from build123d import *

# Parameters (mm, degrees)
F0_W         = 70
F0_H         = 45
F0_W_2       = 20.7
F0_H_2       = 27.2
F0_W_3       = 25.5
F0_H_3       = 32.8
F1_DEPTH     = 2
F2_W         = 70
F2_H         = 45
F2_W_2       = 65
F2_H_2       = 40
F3_DEPTH     = 55
F4_W         = 70
F4_H         = 45
F4_W_2       = 13.2
F4_H_2       = 19.6
F5_DEPTH     = 2.5
F6_W         = 5
F6_H         = 2.5
F7_DEPTH     = 59.501
F8_T1_DEPTH  = 64
F8_T3_DEPTH  = 49.5
F8_T5_DEPTH  = 53.5
F8_S9_W      = 3
F8_S9_H      = 3
F8_T10_DEPTH = 3
F8_S15_W     = 3
F8_S15_H     = 3
F8_T16_DEPTH = 3
F8_S21_W     = 3
F8_S21_H     = 3
F8_T22_DEPTH = 3
F8_S27_W     = 3
F8_S27_H     = 3
F8_T28_DEPTH = 3


# Not quite as in the source:
# - a fillet or chamfer that OpenCascade refuses, or shapes differently, is made with other operations: its cross-section is extruded or revolved along the edge and cut away or added


with BuildPart() as f1:
    # F0 (on Front) → F1 (new body)
    with BuildSketch(Plane.XZ):
        Rectangle(F0_W, F0_H)
        with Locations((17.65, -1.9)):
            Rectangle(F0_W_2, F0_H_2, mode=Mode.SUBTRACT)
        with Locations((-15.25, 0.9)):
            Rectangle(F0_W_3, F0_H_3, mode=Mode.SUBTRACT)
    extrude(amount=F1_DEPTH)

    # F2 (on face) → F3 (join)
    with BuildSketch(Plane.XZ.offset(2)):
        Rectangle(F2_W, F2_H)
        Rectangle(F2_W_2, F2_H_2, mode=Mode.SUBTRACT)
    extrude(amount=F3_DEPTH)

    # F4 (on face) → F5 (join)
    with BuildSketch(Plane.XZ.offset(57)):
        Rectangle(F4_W, F4_H)
        Rectangle(F4_W_2, F4_H_2, mode=Mode.SUBTRACT)
    extrude(amount=F5_DEPTH)

    # F6 (on face) → F7 (cut, through all)
    with BuildSketch(Plane(origin=(0, 0, 0), x_dir=(-1, 0, 0), z_dir=(0, 1, 0))):
        with Locations((-30, -18.75)):
            Rectangle(F6_W, F6_H)
        with Locations((30, -18.75)):
            Rectangle(F6_W, F6_H)
    extrude(amount=-F7_DEPTH, mode=Mode.SUBTRACT)

    # F8: fillet of radius 3 on 8 edges, made by hand

    # F8_s2 → F8_t1 (cut)
    with BuildSketch(Plane.YZ.offset(-32)):
        with BuildLine():
            ThreePointArc((-56.5, 22.5), (-58.6213203436, 21.6213203436), (-59.5, 19.5))
            Line((-59.5, 19.5), (-59.5, 22.5))
            Line((-59.5, 22.5), (-56.5, 22.5))
        make_face()
        with BuildLine():
            ThreePointArc((-3, 22.5), (-0.8786796564, 21.6213203436), (0, 19.5))
            Line((0, 19.5), (0, 22.5))
            Line((0, 22.5), (-3, 22.5))
        make_face()
    extrude(amount=F8_T1_DEPTH, mode=Mode.SUBTRACT)

    # F8_s4 → F8_t3 (cut)
    with BuildSketch(Plane.XY.offset(-30)):
        with BuildLine():
            ThreePointArc((32, -59.5), (34.1213203436, -58.6213203436), (35, -56.5))
            Line((35, -56.5), (35, -59.5))
            Line((35, -59.5), (32, -59.5))
        make_face()
        with BuildLine():
            ThreePointArc((-35, -56.5), (-34.1213203436, -58.6213203436), (-32, -59.5))
            Line((-32, -59.5), (-35, -59.5))
            Line((-35, -59.5), (-35, -56.5))
        make_face()
        with BuildLine():
            ThreePointArc((32, 0), (34.1213203436, -0.8786796564), (35, -3))
            Line((35, -3), (35, 0))
            Line((35, 0), (32, 0))
        make_face()
        with BuildLine():
            ThreePointArc((-32, 0), (-34.1213203436, -0.8786796564), (-35, -3))
            Line((-35, -3), (-35, 0))
            Line((-35, 0), (-32, 0))
        make_face()
    extrude(amount=F8_T3_DEPTH, mode=Mode.SUBTRACT)

    # F8_s6 → F8_t5 (cut)
    with BuildSketch(Plane.XZ.offset(3)):
        with BuildLine():
            ThreePointArc((32, 22.5), (34.1213203436, 21.6213203436), (35, 19.5))
            Line((35, 19.5), (35, 22.5))
            Line((35, 22.5), (32, 22.5))
        make_face()
        with BuildLine():
            ThreePointArc((-32, 22.5), (-34.1213203436, 21.6213203436), (-35, 19.5))
            Line((-35, 19.5), (-35, 22.5))
            Line((-35, 22.5), (-32, 22.5))
        make_face()
    extrude(amount=F8_T5_DEPTH, mode=Mode.SUBTRACT)


with BuildPart() as f8_tool8:
    # F8_s9 → F8_t10 (new body)
    with BuildSketch(Plane.XY.offset(19.5)):
        with Locations((33.5, -58)):
            Rectangle(F8_S9_W, F8_S9_H)
    extrude(amount=F8_T10_DEPTH)

    # F8_s11 → F8_t12 (revolve, cut)
    with BuildSketch(Plane(origin=(32, -56.5, 19.5), x_dir=(-0.7071067812, 0.7071067812, 0), z_dir=(0.7071067812, 0.7071067812, 0))):
        with BuildLine():
            ThreePointArc((0, -3), (3, 0), (0, 3))
            Line((0, 3), (0, -3))
        make_face()
    revolve(axis=Axis((32, -56.5, 19.5), (0, 0, 1)), mode=Mode.SUBTRACT)


with BuildPart() as f1_1:
    add(f1.part)

    # F8_t7: cut F8_tool8
    add(f8_tool8.part, mode=Mode.SUBTRACT)


with BuildPart() as f8_tool14:
    # F8_s15 → F8_t16 (new body)
    with BuildSketch(Plane.XY.offset(19.5)):
        with Locations((-33.5, -58)):
            Rectangle(F8_S15_W, F8_S15_H)
    extrude(amount=F8_T16_DEPTH)

    # F8_s17 → F8_t18 (revolve, cut)
    with BuildSketch(Plane(origin=(-32, -56.5, 19.5), x_dir=(0.7071067812, 0.7071067812, 0), z_dir=(0.7071067812, -0.7071067812, 0))):
        with BuildLine():
            ThreePointArc((0, -3), (3, 0), (0, 3))
            Line((0, 3), (0, -3))
        make_face()
    revolve(axis=Axis((-32, -56.5, 19.5), (0, 0, 1)), mode=Mode.SUBTRACT)


with BuildPart() as f1_2:
    add(f1_1.part)

    # F8_t13: cut F8_tool14
    add(f8_tool14.part, mode=Mode.SUBTRACT)


with BuildPart() as f8_tool20:
    # F8_s21 → F8_t22 (new body)
    with BuildSketch(Plane.XY.offset(19.5)):
        with Locations((33.5, -1.5)):
            Rectangle(F8_S21_W, F8_S21_H)
    extrude(amount=F8_T22_DEPTH)

    # F8_s23 → F8_t24 (revolve, cut)
    with BuildSketch(Plane(origin=(32, -3, 19.5), x_dir=(-0.7071067812, -0.7071067812, 0), z_dir=(-0.7071067812, 0.7071067812, 0))):
        with BuildLine():
            ThreePointArc((0, -3), (3, 0), (0, 3))
            Line((0, 3), (0, -3))
        make_face()
    revolve(axis=Axis((32, -3, 19.5), (0, 0, 1)), mode=Mode.SUBTRACT)


with BuildPart() as f1_3:
    add(f1_2.part)

    # F8_t19: cut F8_tool20
    add(f8_tool20.part, mode=Mode.SUBTRACT)


with BuildPart() as f8_tool26:
    # F8_s27 → F8_t28 (new body)
    with BuildSketch(Plane.XY.offset(19.5)):
        with Locations((-33.5, -1.5)):
            Rectangle(F8_S27_W, F8_S27_H)
    extrude(amount=F8_T28_DEPTH)

    # F8_s29 → F8_t30 (revolve, cut)
    with BuildSketch(Plane(origin=(-32, -3, 19.5), x_dir=(0.7071067812, -0.7071067812, 0), z_dir=(-0.7071067812, -0.7071067812, 0))):
        with BuildLine():
            ThreePointArc((0, -3), (3, 0), (0, 3))
            Line((0, 3), (0, -3))
        make_face()
    revolve(axis=Axis((-32, -3, 19.5), (0, 0, 1)), mode=Mode.SUBTRACT)


with BuildPart() as f1_4:
    add(f1_3.part)

    # F8_t25: cut F8_tool26
    add(f8_tool26.part, mode=Mode.SUBTRACT)


solid = f1_4.part
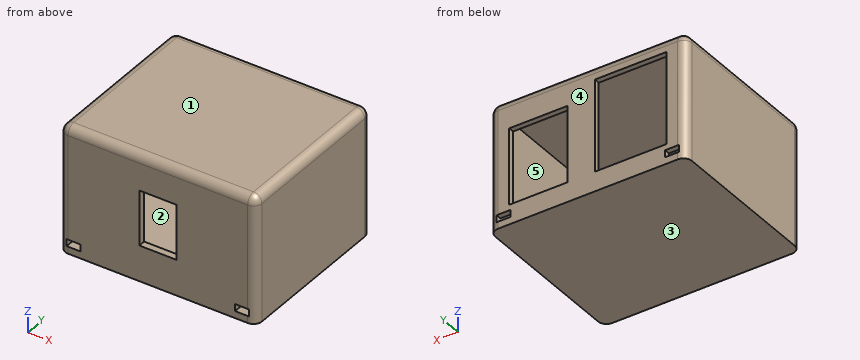
Work out the finished part from the listing and answer in its coordinate system (mm). Face numbers are marked on the shaded views. A direction names the side the tool comes from. Coordinates: 2 decimals unless noted, no trailing zeros. Loops run counter-clockwise (first coordinate to the right, second up) from the corner with the lowest first, then second, coordinate; pieces in that order, holes last. Notation, with made-up numbers: (14, -22) -> (29, -22) arc R16 cw to (29, 6) -> close; hole circle Ø8 at (-19.5, 17). An arc over 180 degrees is marked (long way). Write each question's results on one line, items separated by ' | '. Start each with the question number.
1) The mould has two halves that part along Z. Classify the marked faces 3, 4 and 5: pulls with the +Z half, pulls with the -Z half, needs draft (parallel to the pull), parting line crosses it, or undercut.
2) For the marked faces 1 and 2, determine the directions among +Z, -Z, +X, -X, +Y, -Y from which every point of the face is accessible in a straight line to the end or side of a thin tool.
3) Find section B-B on y = -17.5. Determine the outline of the cut face in (x, z).
4) Flat-ended cylindrical pins translate along their axes: P1, Ø1.2, axis at y = -59, z = -18.5, coming from the +X side; P2, Ø0.6, axis at x = 14.5, y = -1, coming from the +Z side; P3, Ø1.6, axis at y = -1.5, z = 8, coming from the +X side. Find the tip coordinate at first contact, or state that the pin passes through.
5) Find section C-C on z = -11. Determine the outline of the cut face in (x, y), then the cut area to 3 significant figures.
6) Consider line 1 along X through (y, z) = (-21, -7); line 2 along Y through (x, z) = (10, 13.5); line 3 along Z through (x, y) = (15, -36). Determine where each line is inside the solid, lowest interval first.
7) Find section A-A on z = 5.5. Determine the outline of the cut face in (x, y).
8) Find section D-D on x = -15.5. Determine the outline of the cut face in (y, z), then the cut area to 3 significant figures.
Response values:
1) face 3: pulls with the -Z half | face 4: needs draft | face 5: undercut
2) face 1: +Z, +X, -X, +Y, -Y | face 2: none
3) outline: (-35, -22.5) -> (35, -22.5) -> (35, 19.5) arc R3 ccw to (32, 22.5) -> (-32, 22.5) arc R3 ccw to (-35, 19.5) -> close; hole (-32.5, -20) -> (32.5, -20) -> (32.5, 20) -> (-32.5, 20) -> close
4) P1: stops at x = 34.32 | P2: stops at z = 21.97 | P3: stops at x = 34.92
5) outline: (-35, -56.5) arc R3 ccw to (-32, -59.5) -> (32, -59.5) arc R3 ccw to (35, -56.5) -> (35, -3) arc R3 ccw to (32, 0) -> (28, 0) -> (28, -2) -> (32.5, -2) -> (32.5, -57) -> (-32.5, -57) -> (-32.5, -2) -> (-28, -2) -> (-28, 0) -> (-32, 0) arc R3 ccw to (-35, -3) -> close; (-2.5, -2) -> (7.3, -2) -> (7.3, 0) -> (-2.5, 0) -> close | area: 490 mm^2
6) line 1: x = -35 to -32.5, 32.5 to 35 | line 2: y = -59.5 to -57, -2 to 0 | line 3: z = -22.5 to -20, 20 to 22.5
7) outline: (-35, -56.5) arc R3 ccw to (-32, -59.5) -> (-6.6, -59.5) -> (-6.6, -57) -> (-32.5, -57) -> (-32.5, -2) -> (-28, -2) -> (-28, 0) -> (-32, 0) arc R3 ccw to (-35, -3) -> close; (-2.5, -2) -> (7.3, -2) -> (7.3, 0) -> (-2.5, 0) -> close; (6.6, -59.5) -> (32, -59.5) arc R3 ccw to (35, -56.5) -> (35, -3) arc R3 ccw to (32, 0) -> (28, 0) -> (28, -2) -> (32.5, -2) -> (32.5, -57) -> (6.6, -57) -> close
8) outline: (-59.5, -22.5) -> (0, -22.5) -> (0, -15.5) -> (-2, -15.5) -> (-2, -20) -> (-57, -20) -> (-57, 20) -> (-2, 20) -> (-2, 17.3) -> (0, 17.3) -> (0, 19.5) arc R3 ccw to (-3, 22.5) -> (-56.5, 22.5) arc R3 ccw to (-59.5, 19.5) -> close | area: 408 mm^2
